from build123d import *

# Parameters (mm, degrees)
SKETCH1_R           = 5
BOSS_EXTRUDE1_DEPTH = 15
CUT_EXTRUDE1_DEPTH  = 15


with BuildPart() as part:
    # Sketch1 → Boss-Extrude1 (new body)
    with BuildSketch(Plane(origin=(0, 0, 0), x_dir=(0, 0, -1), z_dir=(1, 0, 0))):
        with BuildLine():
            Line((-42.152698982, 21.985337207), (137.847301018, 21.985337207))
            add(Edge.make_bspline(
                [(137.847301018, 21.985337207), (197.847301018, 1.985337207), (137.847301018, -18.014662793)],
                knots=[0, 0, 0, 1, 1, 1], degree=2))
            Line((137.847301018, -18.014662793), (-42.152698982, -18.014662793))
            add(Edge.make_bspline(
                [(-42.152698982, 21.985337207), (-102.152698982, 1.985337207), (-42.152698982, -18.014662793)],
                knots=[0, 0, 0, 1, 1, 1], degree=2))
        make_face()
        with Locations((-57.152698982, 1.985337207)):
            Circle(SKETCH1_R, mode=Mode.SUBTRACT)
        with Locations((152.847301018, 1.985337207)):
            Circle(SKETCH1_R, mode=Mode.SUBTRACT)
    extrude(amount=BOSS_EXTRUDE1_DEPTH)

    # Sketch3 → Cut-Extrude1 (cut)
    with BuildSketch(Plane(origin=(15, 0, 0), x_dir=(0, 0, -1), z_dir=(1, 0, 0))):
        with BuildLine():
            Line((-53.152698982, 10.985337207), (-61.152698982, 10.985337207))
            ThreePointArc((-61.152698982, 10.985337207), (-61.859805763, 10.692443988), (-62.152698982, 9.985337207))
            Line((-62.152698982, 9.985337207), (-62.152698982, -6.014662793))
            ThreePointArc((-62.152698982, -6.014662793), (-61.859805763, -6.721769574), (-61.152698982, -7.014662793))
            Line((-61.152698982, -7.014662793), (-53.152698982, -7.014662793))
            ThreePointArc((-53.152698982, -7.014662793), (-52.4455922, -6.721769574), (-52.152698982, -6.014662793))
            Line((-52.152698982, -6.014662793), (-52.152698982, 9.985337207))
            ThreePointArc((-52.152698982, 9.985337207), (-52.4455922, 10.692443988), (-53.152698982, 10.985337207))
        make_face()
    extrude(amount=-CUT_EXTRUDE1_DEPTH, mode=Mode.SUBTRACT)


solid = part.part
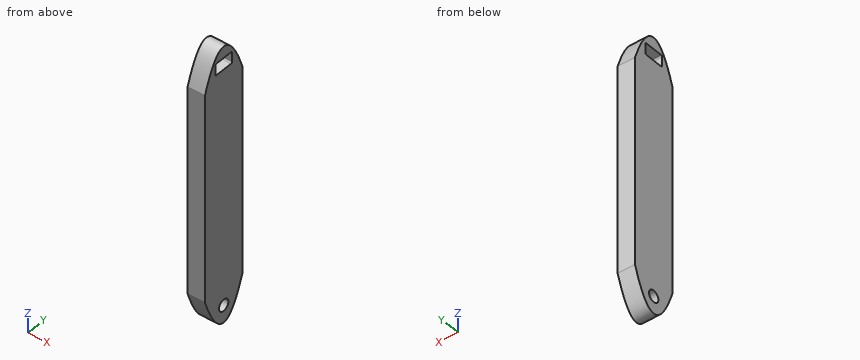
CAD build for the part. Positions are in the model's coordinates, mm. Coordinates: 2 decimals unless noted, no trailing zeros. Write item = value, one per line. Start each with the question number.
Q1. Cut at A-A, the plane x = 9.25. Give the number of separate pieces and of enclosed holes in the cut face, then the cut area to 3 significant figures.
Q2. Flat gauge pins, fed straight in: pin 1 Ø1.5 at (x, y) = (3.5, -8) entering from +Z; pin 2 Ø1 at (x, y) = (5.5, 12) entering from +Z; pin 3 Ø2.5 at (x, z) = (7, 58) entering from +Y. Where does each tip first touch, or does it go through?
Q3. Drill centre lines: L1, parallel to Z at x = 4.5, y = 2; L2, parallel to Z at x = 9.5, y = 3; L3, parallel to Y at x = 13, z = 60.5. Where is each one in solid material? Low to high.
Computed:
q1.separate_pieces = 1
q1.enclosed_holes = 2
q1.area = 8,540 mm²
q2.pin_1 = 65.76
q2.pin_2 = 65.36
q2.pin_3 = 16.32
q3.L1 = -167.85 to -157.85, -147.85 to 52.15, 62.15 to 72.15
q3.L2 = -167.77 to -157.74, -147.95 to 52.15, 62.15 to 72.08
q3.L3 = -10.48 to -7.01, 10.99 to 14.45
